Job drawing, mm, ordinate dimensions from the low corner. One solid piece. A direction names the side the tool comes from. Coordinates: 2 decimals unless noted, no trailing zeros. Write each loop counter-clockwise with the first axis right and the second up, starting at its lowest first coordinate (ties: lowest second). Pieces come first, ordered by that corner, then holes. Notation, with made-up numbers: (-12.5, -37.5) - (37.5, -37.5) arc R25 ccw to (37.5, -25.5) - close; hole circle Ø11 at (-31, 65.5). An arc over 180 degrees is marked (long way). Put each result on its own line as item: value. Start each with the question number.
1. Saw through at B-B, the plane y = 15.75. Write the cut outline in (x, z).
2. Drop flat-ended pins along their axis: P1, Ø11, axis at x = 47, z = 21.5, coming from the +Y side; P2, Ø2, axis at x = 26, y = 9.5, coming from the +Z side; P3, Ø12, axis at x = 31.5, z = 18, coming from the +Y side. Give the stop position or say it passes through.
3. Saw through at C-C, the plane x = 52. Write the cut outline in (y, z), plus the area to 3 significant figures.
4. Saw through at D-D, the plane z = 3. Write the cut outline in (x, y).
5. Which spindle directions (+Z, -Z, +X, -X, +Y, -Y) get a long thin tool onto all of the face, cutting with end or side? Do the marked faces 1 and 2. Say none if no direction does.
6. Drill centre lines: L1, parallel to Y at x = 51.5, z = 22; L2, parallel to X at y = 15, z = 17.5; L3, parallel to Z at x = 36.5, y = 13.25. Where is each one in solid material? Low to high. Write a range as from..to.
7. Saw through at A-A, the plane z = 19.75. Write the cut outline in (x, y).
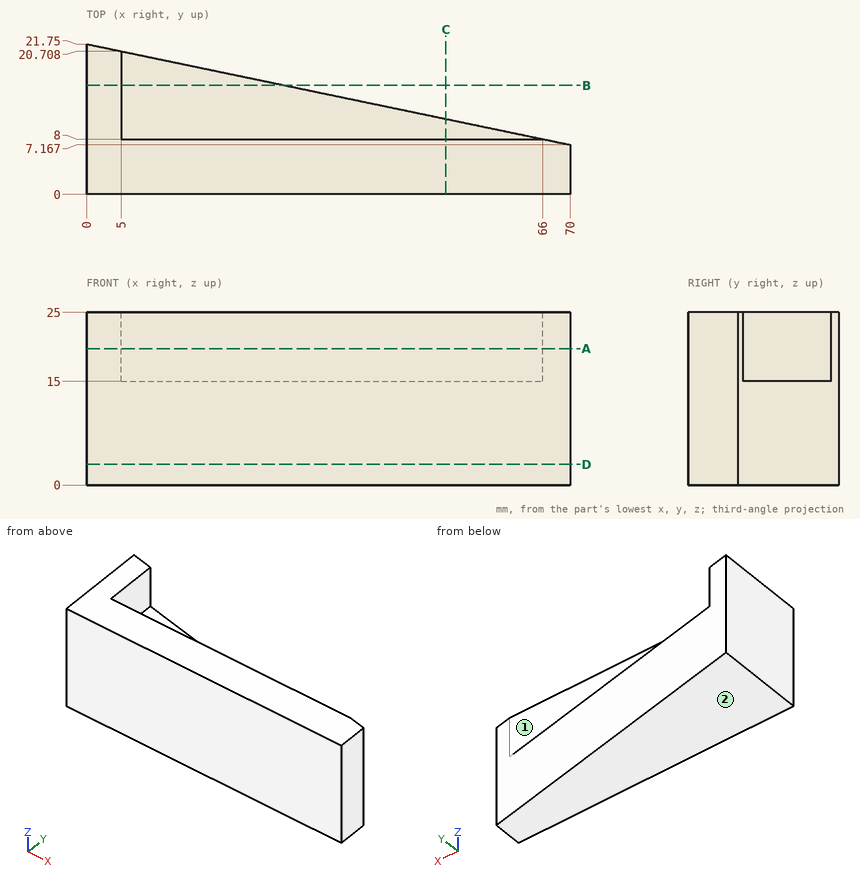
Final values:
1. outline: (0, 0) - (28.8, 0) - (28.8, 15) - (5, 15) - (5, 25) - (0, 25) - close
2. P1: stops at y = 8
2. P2: stops at z = 15
2. P3: stops at y = 16.27
3. outline: (0, 0) - (10.92, 0) - (10.92, 15) - (8, 15) - (8, 25) - (0, 25) - close
3. area: 244 mm²
4. outline: (0, 0) - (70, 0) - (70, 7.17) - (0, 21.75) - close
5. face 1: +Z, +X, +Y
5. face 2: -Z, +X, -X, +Y, -Y
6. L1: y = 0..8
6. L2: x = 0..5
6. L3: z = 0..15
7. outline: (0, 0) - (70, 0) - (70, 7.17) - (66, 8) - (5, 8) - (5, 20.71) - (0, 21.75) - close
